The listing builds one solid part. Answer for the finished solid, in the listing's coordinates (mm). Face numbers are marked on the shaded views. Round coordinates to 2 decimals unless told otherwise and drop trailing zeros. Write each loop counter-clockwise with the first axis right and the second up, starting at its lowest first coordinate (ties: lowest second). Pieces come first, ordered by that corner, then holes.
from build123d import *

# Parameters (mm, degrees)
BOSS_1_DEPTH = 2.95
S_HOLE2_R    = 1.25
HOLE_2_DEPTH = 3.2
S_HOLE3_R    = 1.25
HOLE_3_DEPTH = 3.2
S_HOLE4_R    = 1.25
HOLE_4_DEPTH = 3.2
S_HOLE5_R    = 1.25
HOLE_5_DEPTH = 3.2
S_HOLE6_R    = 1.25
HOLE_6_DEPTH = 3.2


with BuildPart() as part:
    # S_prism1 → Boss_1 (new body)
    with BuildSketch(Plane(origin=(34, 0, 0), x_dir=(0, 0, -1), z_dir=(1, 0, 0))):
        with BuildLine():
            Line((-17.55, -18.3), (-17.55, 18.3))
            ThreePointArc((-17.55, 18.3), (-20.0835, 24.4165), (-26.2, 26.95))
            Line((-26.2, 26.95), (-37.8, 26.95))
            ThreePointArc((-37.8, 26.95), (-43.9165, 24.4165), (-46.45, 18.3))
            Line((-46.45, 18.3), (-46.45, -18.3))
            ThreePointArc((-46.45, -18.3), (-43.9165, -24.4165), (-37.8, -26.95))
            Line((-37.8, -26.95), (-26.2, -26.95))
            ThreePointArc((-26.2, -26.95), (-20.0835, -24.4165), (-17.55, -18.3))
        make_face()
    extrude(amount=BOSS_1_DEPTH)

    # S_hole2 → Hole_2 (cut)
    with BuildSketch(Plane(origin=(33.9, 0, 0), x_dir=(0, 0, -1), z_dir=(1, 0, 0))):
        with Locations((-25, -9)):
            Circle(S_HOLE2_R)
    extrude(amount=HOLE_2_DEPTH, mode=Mode.SUBTRACT)

    # S_hole3 → Hole_3 (cut)
    with BuildSketch(Plane(origin=(33.9, 0, 0), x_dir=(0, 0, -1), z_dir=(1, 0, 0))):
        with Locations((-25, -4.5)):
            Circle(S_HOLE3_R)
    extrude(amount=HOLE_3_DEPTH, mode=Mode.SUBTRACT)

    # S_hole4 → Hole_4 (cut)
    with BuildSketch(Plane(origin=(33.9, 0, 0), x_dir=(0, 0, -1), z_dir=(1, 0, 0))):
        with Locations((-25, 0)):
            Circle(S_HOLE4_R)
    extrude(amount=HOLE_4_DEPTH, mode=Mode.SUBTRACT)

    # S_hole5 → Hole_5 (cut)
    with BuildSketch(Plane(origin=(33.9, 0, 0), x_dir=(0, 0, -1), z_dir=(1, 0, 0))):
        with Locations((-25, 4.5)):
            Circle(S_HOLE5_R)
    extrude(amount=HOLE_5_DEPTH, mode=Mode.SUBTRACT)

    # S_hole6 → Hole_6 (cut)
    with BuildSketch(Plane(origin=(33.9, 0, 0), x_dir=(0, 0, -1), z_dir=(1, 0, 0))):
        with Locations((-25, 9)):
            Circle(S_HOLE6_R)
    extrude(amount=HOLE_6_DEPTH, mode=Mode.SUBTRACT)


solid = part.part
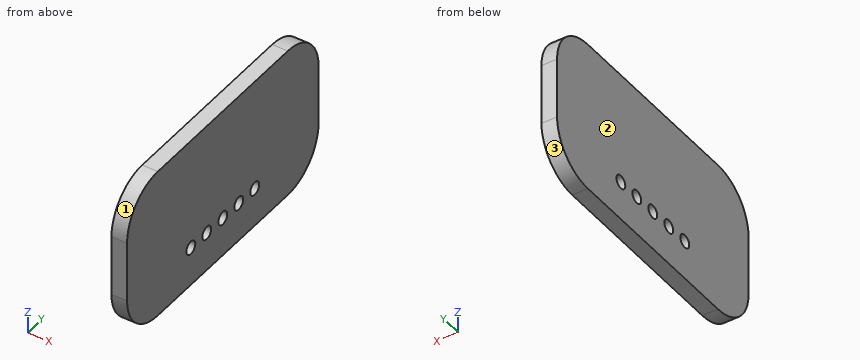
1. Section A-A on x = 34.45 is taken. Determine the outline of the cut face in (y, z).
Geometry says:
outline: (-26.95, 26.2) arc R8.65 ccw to (-18.3, 17.55) - (18.3, 17.55) arc R8.65 ccw to (26.95, 26.2) - (26.95, 37.8) arc R8.65 ccw to (18.3, 46.45) - (-18.3, 46.45) arc R8.65 ccw to (-26.95, 37.8) - close; hole circle Ø2.5 at (-9, 25); hole circle Ø2.5 at (-4.5, 25); hole circle Ø2.5 at (0, 25); hole circle Ø2.5 at (4.5, 25); hole circle Ø2.5 at (9, 25)
2. Section B-B on y = -4 is taken. Determine the outline of the cut face in (x, z), plus the area to 3 significant figures.
Geometry says:
outline: (34, 17.55) - (36.95, 17.55) - (36.95, 23.85) - (34, 23.85) - close; (34, 26.15) - (36.95, 26.15) - (36.95, 46.45) - (34, 46.45) - close
area: 78.5 mm2
3. Section D-D on y = -22 is taken. Determine the outline of the cut face in (x, z).
Geometry says:
outline: (34, 18.38) - (36.95, 18.38) - (36.95, 45.62) - (34, 45.62) - close
4. For a pull along Y with two mould halves and no side action, classify the marked faces 1, 2 and 3 as released by +Y, released by -Y, zero draft, split by the parting line, or undercut.
Geometry says:
face 1: released by -Y
face 2: zero draft
face 3: released by +Y
5. Section C-C on z = 25 is taken. Determine the outline of the cut face in (x, y).
Geometry says:
outline: (34, -26.87) - (36.95, -26.87) - (36.95, -10.25) - (34, -10.25) - close; (34, -7.75) - (36.95, -7.75) - (36.95, -5.75) - (34, -5.75) - close; (34, -3.25) - (36.95, -3.25) - (36.95, -1.25) - (34, -1.25) - close; (34, 1.25) - (36.95, 1.25) - (36.95, 3.25) - (34, 3.25) - close; (34, 5.75) - (36.95, 5.75) - (36.95, 7.75) - (34, 7.75) - close; (34, 10.25) - (36.95, 10.25) - (36.95, 26.87) - (34, 26.87) - close
6. Straight lines are drawn through the part: line 1 along Y through (x, z) = (35.5, 25); line 2 along Z through (x, y) = (34.6, 4.5); line 3 along Y through (x, z) = (34.9, 25.5). For each, find the intervals that lie inside material, in ascending order.
Geometry says:
line 1: y = -26.87 to -10.25, -7.75 to -5.75, -3.25 to -1.25, 1.25 to 3.25, 5.75 to 7.75, 10.25 to 26.87
line 2: z = 17.55 to 23.75, 26.25 to 46.45
line 3: y = -26.92 to -10.15, -7.85 to -5.65, -3.35 to -1.15, 1.15 to 3.35, 5.65 to 7.85, 10.15 to 26.92
